from build123d import *

# Parameters (mm, degrees)
SKETCH1_W           = 500
SKETCH1_H           = 500
BOSS_EXTRUDE1_DEPTH = 100
SKETCH2_W           = 300
SKETCH2_H           = 300
BOSS_EXTRUDE2_DEPTH = 100
SKETCH3_W           = 200
SKETCH3_H           = 200
BOSS_EXTRUDE3_DEPTH = 100
SKETCH4_R           = 60
BOSS_EXTRUDE4_DEPTH = 455
SKETCH5_R           = 36.5
BOSS_EXTRUDE5_DEPTH = 45


with BuildPart() as part:
    # Sketch1 → Boss-Extrude1 (new body)
    with BuildSketch(Plane(origin=(0, 0, 0), x_dir=(1, 0, 0), z_dir=(0, 1, 0))):
        Rectangle(SKETCH1_W, SKETCH1_H)
    extrude(amount=BOSS_EXTRUDE1_DEPTH)

    # Sketch2 → Boss-Extrude2 (add)
    with BuildSketch(Plane(origin=(0, 100, 0), x_dir=(1, 0, 0), z_dir=(0, 1, 0))):
        Rectangle(SKETCH2_W, SKETCH2_H)
    extrude(amount=BOSS_EXTRUDE2_DEPTH)

    # Sketch3 → Boss-Extrude3 (add)
    with BuildSketch(Plane(origin=(0, 200, 0), x_dir=(1, 0, 0), z_dir=(0, 1, 0))):
        Rectangle(SKETCH3_W, SKETCH3_H)
    extrude(amount=BOSS_EXTRUDE3_DEPTH)

    # Sketch4 → Boss-Extrude4 (add)
    with BuildSketch(Plane(origin=(0, 300, 0), x_dir=(1, 0, 0), z_dir=(0, 1, 0))):
        with Locations(Location((0, 0, 0), (0, 0, 90))):
            Circle(SKETCH4_R)
    extrude(amount=BOSS_EXTRUDE4_DEPTH)

    # Sketch5 → Boss-Extrude5 (add)
    with BuildSketch(Plane(origin=(0, 755, 0), x_dir=(1, 0, 0), z_dir=(0, 1, 0))):
        with Locations(Location((0, 0, 0), (0, 0, 90))):
            Circle(SKETCH5_R)
    extrude(amount=BOSS_EXTRUDE5_DEPTH)


solid = part.part
Source: CAD feature listing. Evaluate the final solid. Frame: model axes, mm. A direction names the side the tool comes from. Give positions to 0.01 mm unless a question says otherwise; leave off trailing zeros. Order: outer loops, then holes, each group sorted by start corner. A loop starts at its lowest first (then second) coordinate and runs counter-clockwise, first axis right, second up. Notation, with made-up numbers: (77.5, 30) -> (84.5, 30) arc R34 ccw to (84.5, 61) -> close; hole circle Ø6 at (72.25, -7.75). An arc over 180 degrees is marked (long way). Use a Markdown table: item, result.
1) Ray query, line 1 along Z through (x, y) = (-149, 164); line 2 along X through (y, z) = (240.5, 45.5); line 3 along Y through (x, z) = (-55, -108). Return the intervals inside material, ascending. Write a range as [from, to].
Answer list:
| item | result |
|---|---|
| line 1 | [-150, 150] |
| line 2 | [-100, 100] |
| line 3 | [0, 200] |
2) Section query C-C, the plane y = 232. Return the cut outline in (x, z), then the cut area to 3 significant figures.
Answer list:
| item | result |
|---|---|
| outline | (-100, -100) -> (100, -100) -> (100, 100) -> (-100, 100) -> close |
| area | 40,000 mm² |
3) Contact query for flat-ended pins moving along their axis: P1, Ø8, axis at x = -32.5, y = 316, coming from the -Z side; P2, Ø4, axis at y = 122.5, z = 46.5, coming from the +X side; P3, Ø4, axis at y = 106.5, z = 3.5, coming from the -X side. Output: stop coordinate, or through.
Answer list:
| item | result |
|---|---|
| P1 | z = -52.8 |
| P2 | x = 150 |
| P3 | x = -150 |
4) Section query A-A, the plane x = 0. Return the cut outline in (y, z), then the cut area to 3 significant figures.
Answer list:
| item | result |
|---|---|
| outline | (0, -250) -> (100, -250) -> (100, -150) -> (200, -150) -> (200, -100) -> (300, -100) -> (300, -60) -> (755, -60) -> (755, -36.5) -> (800, -36.5) -> (800, 36.5) -> (755, 36.5) -> (755, 60) -> (300, 60) -> (300, 100) -> (200, 100) -> (200, 150) -> (100, 150) -> (100, 250) -> (0, 250) -> close |
| area | 158,000 mm² |
5) Reachability of faces 1 (the flat face through (-150, 149, 2)), 2 (the flat face through (26, 755, -26)), 3 (the flat face through (150, 149, 2)) from +Z, -Z, +X, -X, +Y, -Y: full face, straight path, thin tool, end or side. Return the list, or none.
Answer list:
| item | result |
|---|---|
| face 1 | +Z, -Z, -X, +Y |
| face 2 | +Y |
| face 3 | +Z, -Z, +X, +Y |
6) Section query B-B, the plane z = 0. Return the cut outline in (x, y), then the cut area to 3 significant figures.
Answer list:
| item | result |
|---|---|
| outline | (-250, 0) -> (250, 0) -> (250, 100) -> (150, 100) -> (150, 200) -> (100, 200) -> (100, 300) -> (60, 300) -> (60, 755) -> (36.5, 755) -> (36.5, 800) -> (-36.5, 800) -> (-36.5, 755) -> (-60, 755) -> (-60, 300) -> (-100, 300) -> (-100, 200) -> (-150, 200) -> (-150, 100) -> (-250, 100) -> close |
| area | 158,000 mm² |
7) Section query D-D, the plane z = -110. Return the cut outline in (x, y).
Answer list:
| item | result |
|---|---|
| outline | (-250, 0) -> (250, 0) -> (250, 100) -> (150, 100) -> (150, 200) -> (-150, 200) -> (-150, 100) -> (-250, 100) -> close |
